Read the model definition and answer for the solid it produces. Units are mm, in the model's axes. Give positions to 0.01 mm unless a question says otherwise; leave off trailing zeros. Order: outer loops, then holes, each group sorted by start corner. A loop starts at its lowest first (then second) coordinate and runs counter-clockwise, first axis right, second up.
Item 1: Given pin 1 Ø3 at (y, z) = (52, 3) entering from -X; pin 2 Ø3 at (y, z) = (39, 1.5) entering from +X; pin 3 Ø2.5 at (x, y) = (50, 94.5) entering from -Z, each flat-ended and moving along its own axis, determine where each tip first touches the part or whether it passes through.
Item 2: Find the intervals of material crossed by line 1 along Y through (x, z) = (-114, 1.55); line 2 along Y through (x, z) = (-114, 8); line 3 along X through (y, z) = (56.5, 4), in increasing order.
Item 3: A cutting plane is placed at B-B (y = 75). Write down the section's boundary in (x, z), plus the area to 3 significant figures.
Item 4: A cutting plane is placed at C-C (z = 6). Write down the section's boundary in (x, y), plus the area to 3 significant figures.
Item 5: A cutting plane is placed at A-A (x = 26.5). Write down the section's boundary in (y, z).
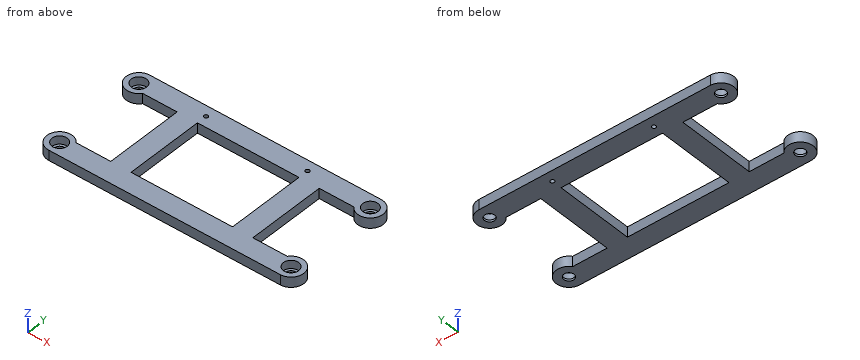
from build123d import *

# Parameters (mm, degrees)
SKETCH_1_R          = 5
SKETCH_1_W          = 100
SKETCH_1_H          = 77
EXTRUDE_1_DEPTH     = 10
SKETCH_3_R          = 7.5
CUT_EXTRUDE_1_DEPTH = 8
CUT_EXTRUDE_2_REACH = 166.385
SKETCH_5_R          = 2


with BuildPart() as part:
    # 草图1 → 凸台-拉伸1 (new body)
    with BuildSketch(Plane.XY):
        with BuildLine():
            Line((-104, 84.5), (-70, 84.5))
            Line((-70, 84.5), (-70, 7.5))
            Line((-70, 7.5), (-104, 7.5))
            ThreePointArc((-104, 7.5), (-125.180339887, 5.590169944), (-114, -12.5))
            Line((-114, -12.5), (114, -12.5))
            ThreePointArc((114, -12.5), (125.180339887, 5.590169944), (104, 7.5))
            Line((104, 7.5), (70, 7.5))
            Line((70, 7.5), (70, 84.5))
            Line((70, 84.5), (104, 84.5))
            ThreePointArc((104, 84.5), (125.180339887, 86.409830056), (114, 104.5))
            Line((114, 104.5), (64, 104.5))
            Line((64, 104.5), (-64, 104.5))
            Line((-64, 104.5), (-114, 104.5))
            ThreePointArc((-114, 104.5), (-125.180339887, 86.409830056), (-104, 84.5))
        make_face()
        with Locations((-114, 0)):
            Circle(SKETCH_1_R, mode=Mode.SUBTRACT)
        with Locations((-114, 92)):
            Circle(SKETCH_1_R, mode=Mode.SUBTRACT)
        with Locations(Location((114, 92, 0), (0, 0, 180))):
            Circle(SKETCH_1_R, mode=Mode.SUBTRACT)
        with Locations(Location((114, 0, 0), (0, 0, 180))):
            Circle(SKETCH_1_R, mode=Mode.SUBTRACT)
        with Locations((0, 46)):
            Rectangle(SKETCH_1_W, SKETCH_1_H, mode=Mode.SUBTRACT)
    extrude(amount=EXTRUDE_1_DEPTH)

    # 草图3 → 切除-拉伸1 (cut)
    with BuildSketch(Plane.XY.offset(10)):
        with Locations((-114, 92)):
            Circle(SKETCH_3_R)
        with Locations((-114, 0)):
            Circle(SKETCH_3_R)
        with Locations(Location((114, 0, 0), (0, 0, 180))):
            Circle(SKETCH_3_R)
        with Locations(Location((114, 92, 0), (0, 0, 180))):
            Circle(SKETCH_3_R)
    extrude(amount=-CUT_EXTRUDE_1_DEPTH, mode=Mode.SUBTRACT)

    # 草图5 → 切除-拉伸2 (cut, up to next)
    with BuildSketch(Plane.XY, mode=Mode.PRIVATE) as cut_extrude_2_sk1:
        with Locations(Location((-50, 94.5, 0), (0, 0, 180))):
            Circle(SKETCH_5_R)
    cut_extrude_2_tool1 = extrude(cut_extrude_2_sk1.sketch, amount=CUT_EXTRUDE_2_REACH, mode=Mode.PRIVATE) & part.part
    # 草图5 → 切除-拉伸2 (cut, up to next)
    with BuildSketch(Plane.XY, mode=Mode.PRIVATE) as cut_extrude_2_sk2:
        with Locations(Location((50, 94.5, 0), (0, 0, 180))):
            Circle(SKETCH_5_R)
    cut_extrude_2_tool2 = extrude(cut_extrude_2_sk2.sketch, amount=CUT_EXTRUDE_2_REACH, mode=Mode.PRIVATE) & part.part
    add(cut_extrude_2_tool1.solids().sort_by_distance((-50, 94.5, 0))[0], mode=Mode.SUBTRACT)
    add(cut_extrude_2_tool2.solids().sort_by_distance((50, 94.5, 0))[0], mode=Mode.SUBTRACT)


solid = part.part
Response values:
1. pin 1: stops at x = -70
1. pin 2: stops at x = 70
1. pin 3: passes through
2. line 1: y = -12.5 to -5, 5 to 12.5, 79.5 to 87, 97 to 104.5
2. line 2: y = -12.5 to -7.5, 7.5 to 12.5, 79.5 to 84.5, 99.5 to 104.5
2. line 3: x = -70 to -50, 50 to 70
3. outline: (-70, 0) - (-50, 0) - (-50, 10) - (-70, 10) - close; (50, 0) - (70, 0) - (70, 10) - (50, 10) - close
3. area: 400 mm2
4. outline: (-114, -12.5) - (114, -12.5) arc R12.5 ccw (long way) to (104, 7.5) - (70, 7.5) - (70, 84.5) - (104, 84.5) arc R12.5 ccw (long way) to (114, 104.5) - (-114, 104.5) arc R12.5 ccw (long way) to (-104, 84.5) - (-70, 84.5) - (-70, 7.5) - (-104, 7.5) arc R12.5 ccw (long way) to start; hole circle Ø15 at (-114, 0); hole circle Ø15 at (-114, 92); hole circle Ø4 at (-50, 94.5); hole (-50, 7.5) - (50, 7.5) - (50, 84.5) - (-50, 84.5) - close; hole circle Ø4 at (50, 94.5); hole circle Ø15 at (114, 0); hole circle Ø15 at (114, 92)
4. area: 12,600 mm2
5. outline: (-12.5, 0) - (7.5, 0) - (7.5, 10) - (-12.5, 10) - close; (84.5, 0) - (104.5, 0) - (104.5, 10) - (84.5, 10) - close
